Autodesk Inventor part; units mm, degrees
ref_plane "YZ Plane" through (0, 0, 0) normal (1, 0, 0) x (0, 1, 0)
ref_plane "XZ Plane" through (0, 0, 0) normal (0, 1, 0) x (-1, 0, 0)
ref_plane "XY Plane" through (0, 0, 0) normal (0, 0, 1) x (1, 0, 0)
sketch "Sketch1" plane through (0, 0, 0) normal (0, 1, 0) x (-1, 0, 0)
  line L0 (0, 0) -> (-100, 0)
  line L1 (-100, 0) -> (-100, -75)
  line L2 (-100, -75) -> (0, -75)
  line L3 (0, -75) -> (0, 0)
  dimension "d0" = 100
  dimension "d1" = 75
extrude "Extrusion1" add sketch "Sketch1" along normal blind 4
sketch "Sketch2" plane through (0, 4, 0) normal (0, 1, 0) x (1, 0, 0)
  line L0 (0, 0) -> (100, 0) construction
  line L1 (100, 0) -> (100, 75) construction
  line L2 (100, 75) -> (0, 75) construction
  line L3 (0, 75) -> (0, 0) construction
  line L4 (4, 71) -> (96, 71)
  line L5 (96, 71) -> (96, 4)
  line L6 (96, 4) -> (4, 4)
  line L7 (4, 4) -> (4, 71)
  line L8 (92, 67) -> (8, 67)
  line L9 (8, 67) -> (8, 8)
  line L10 (8, 8) -> (92, 8)
  line L11 (92, 8) -> (92, 67)
  dimension "d4" = 4
  dimension "d5" = 4
extrude "Extrusion2" add sketch "Sketch2" along normal blind 7
sketch "Sketch3" plane through (0, 4, 0) normal (0, 1, 0) x (1, 0, 0)
  line L0 (100, 75) -> (0, 75) construction
  line L1 (0, 75) -> (0, 0) construction
  line L2 (0, 0) -> (100, 0) construction
  line L3 (100, 0) -> (100, 75) construction
  line L4 (4, 71) -> (96, 71) construction
  line L5 (96, 71) -> (96, 4) construction
  line L6 (96, 4) -> (4, 4) construction
  line L7 (4, 4) -> (4, 71) construction
  line L8 (0, 37.5) -> (100, 37.5) construction
  line L9 (50, 75) -> (50, 0) construction
  line L10 (0, 65.5) -> (4, 65.5)
  line L11 (4, 65.5) -> (4, 71)
  line L12 (4, 71) -> (14, 71)
  line L13 (4, 71) -> (96, 71)
  line L14 (14, 71) -> (14, 75)
  line L15 (14, 75) -> (0, 75)
  line L16 (0, 75) -> (0, 65.5)
  line L17 (0, 57.5) -> (4, 57.5)
  line L18 (4, 57.5) -> (4, 49.5)
  line L19 (4, 71) -> (4, 4)
  line L20 (4, 49.5) -> (0, 49.5)
  line L21 (0, 49.5) -> (0, 57.5)
  line L22 (0, 41.5) -> (4, 41.5)
  line L23 (4, 37.5) -> (4, 41.5)
  line L24 (0, 41.5) -> (0, 37.5)
  line L25 (22, 75) -> (22, 71)
  line L26 (22, 71) -> (30, 71)
  line L27 (30, 71) -> (30, 75)
  line L28 (30, 75) -> (22, 75)
  line L29 (38, 75) -> (38, 71)
  line L30 (38, 71) -> (46, 71)
  line L31 (46, 71) -> (46, 75)
  line L32 (46, 75) -> (38, 75)
  line L33 (0, 9.5) -> (4, 9.5)
  line L34 (4, 9.5) -> (4, 4)
  line L35 (4, 4) -> (14, 4)
  line L36 (14, 4) -> (14, 0)
  line L37 (14, 0) -> (0, 0)
  line L38 (0, 0) -> (0, 9.5)
  line L39 (0, 17.5) -> (4, 17.5)
  line L40 (4, 17.5) -> (4, 25.5)
  line L41 (4, 25.5) -> (0, 25.5)
  line L42 (0, 25.5) -> (0, 17.5)
  line L43 (0, 33.5) -> (4, 33.5)
  line L44 (4, 37.5) -> (4, 33.5)
  line L45 (0, 33.5) -> (0, 37.5)
  line L46 (22, 0) -> (22, 4)
  line L47 (22, 4) -> (30, 4)
  line L48 (30, 4) -> (30, 0)
  line L49 (30, 0) -> (22, 0)
  line L50 (38, 0) -> (38, 4)
  line L51 (38, 4) -> (46, 4)
  line L52 (46, 4) -> (46, 0)
  line L53 (46, 0) -> (38, 0)
  line L54 (100, 75) -> (100, 0) construction
  line L55 (96, 4) -> (96, 71) construction
  line L56 (100, 65.5) -> (96, 65.5)
  line L57 (96, 65.5) -> (96, 71)
  line L58 (96, 71) -> (86, 71)
  line L59 (86, 71) -> (86, 75)
  line L60 (86, 75) -> (100, 75)
  line L61 (100, 75) -> (100, 65.5)
  line L62 (100, 57.5) -> (96, 57.5)
  line L63 (96, 57.5) -> (96, 49.5)
  line L64 (96, 71) -> (96, 4)
  line L65 (96, 49.5) -> (100, 49.5)
  line L66 (100, 49.5) -> (100, 57.5)
  line L67 (100, 41.5) -> (96, 41.5)
  line L68 (96, 37.5) -> (96, 41.5)
  line L69 (100, 41.5) -> (100, 37.5)
  line L70 (78, 75) -> (78, 71)
  line L71 (78, 71) -> (70, 71)
  line L72 (70, 71) -> (70, 75)
  line L73 (70, 75) -> (78, 75)
  line L74 (62, 75) -> (62, 71)
  line L75 (62, 71) -> (54, 71)
  line L76 (54, 71) -> (54, 75)
  line L77 (54, 75) -> (62, 75)
  line L78 (78, 0) -> (78, 4)
  line L79 (70, 4) -> (70, 0)
  line L80 (78, 4) -> (70, 4)
  line L81 (70, 0) -> (78, 0)
  line L82 (54, 4) -> (54, 0)
  line L83 (62, 4) -> (54, 4)
  line L84 (54, 0) -> (62, 0)
  line L85 (62, 0) -> (62, 4)
  line L86 (96, 4) -> (86, 4)
  line L87 (100, 9.5) -> (96, 9.5)
  line L88 (96, 9.5) -> (96, 4)
  line L89 (86, 4) -> (86, 0)
  line L90 (86, 0) -> (100, 0)
  line L91 (96, 17.5) -> (96, 25.5)
  line L92 (100, 17.5) -> (96, 17.5)
  line L93 (96, 25.5) -> (100, 25.5)
  line L94 (96, 37.5) -> (96, 33.5)
  line L95 (100, 33.5) -> (96, 33.5)
  line L96 (100, 33.5) -> (100, 37.5)
  line L97 (100, 25.5) -> (100, 17.5)
  line L98 (100, 0) -> (100, 9.5)
  dimension "d9" = 8
  dimension "d11" = 4
  dimension "d12" = 8
  dimension "d13" = 8
  dimension "d14" = 8
  dimension "d15" = 8
  dimension "d16" = 8
  dimension "d17" = 4
  dimension "d18" = 8
extrude "Extrusion3" cut sketch "Sketch3" against normal up to surface (4 mm away)
properties part number "bottom" material "PBT Plastic Black"
For this review, take the finished solid that the model builds, in its own axes (mm). A direction names the side the tool comes from. Round coordinates to 2 decimals unless told otherwise and drop trailing zeros. Loops run counter-clockwise (first coordinate to the right, second up) from the corner with the lowest first, then second, coordinate; pieces in that order, holes last. Notation, with made-up numbers: (1.25, 67) - (57.25, 67) arc R24 ccw to (57.25, 77) - close; hole circle Ø9 at (69, 82.5). An arc over 180 degrees is marked (long way). Use one line per item in the form item = value.
1) We need section A-A on x = 10.5. Write out the cut boundary in (y, z), then the cut area to 3 significant figures.
Solutions:
outline = (0, -71) - (11, -71) - (11, -67) - (4, -67) - (4, -8) - (11, -8) - (11, -4) - (0, -4) - close
area = 324 mm2
2) We need section C-C on y = 7.75. Write out the cut boundary in (x, z), then the cut area to 3 significant figures.
Solutions:
outline = (4, -71) - (96, -71) - (96, -4) - (4, -4) - close; hole (8, -67) - (92, -67) - (92, -8) - (8, -8) - close
area = 1,210 mm2
3) Mouldability with a two-part tool opening along X and no side actions: class faces 4 (the face through (2, 4, -29)), 5 (the face through (46, 2, -73)) as pulls with the +X half, pulls with the -X half, needs draft (parallel to the pull), parting line crosses it, or undercut.
Solutions:
face_4 = needs draft
face_5 = undercut
4) We need section D-D on z = -22. Write out the cut boundary in (x, y), then the cut area to 3 significant figures.
Solutions:
outline = (4, 0) - (96, 0) - (96, 11) - (92, 11) - (92, 4) - (8, 4) - (8, 11) - (4, 11) - close
area = 424 mm2
5) Tool access review of faces 1 (the face through (51, 7, -67)), 2 (the face through (70, 2, -73)), 3 (the face through (98, 2, -33.5)): name each direction out of +Z, -Z, +X, -X, +Y, -Y from which nothing blocks a thin tool from reaching the whole face with its end or side.
Solutions:
face_1 = +Y
face_2 = -Z, +Y, -Y
face_3 = +X, +Y, -Y
6) Clearance check with flat-ended pins moving along their axes: P1, Ø2, axis at x = 1.5, z = -15.5, coming from the +Y side; P2, Ø1.2, axis at y = 2, z = -3, coming from the +X side; P3, Ø1.2, axis at x = 2, y = 3, coming from the +Z side. State where each tip first meets the part, or that it passes through.
Solutions:
P1 = 4
P2 = 86
P3 = -9.5
7) We need section B-B on z = -12.5. Write out the cut boundary in (x, y), then the cut area to 3 significant figures.
Solutions:
outline = (0, 0) - (100, 0) - (100, 4) - (96, 4) - (96, 11) - (92, 11) - (92, 4) - (8, 4) - (8, 11) - (4, 11) - (4, 4) - (0, 4) - close
area = 456 mm2
8) Wall thickness on probe 1 along Z at (x, y) = (66.5, 9); probe 2 along X at (y, z) = (8, -29); probe 3 along Y at (x, z) = (86.5, -53.5): over which ranges is each line inside the solid? List them lowest first.
Solutions:
probe_1 = -71 to -67, -8 to -4
probe_2 = 4 to 8, 92 to 96
probe_3 = 0 to 4
